Can you work these out from the model? Positions are in its coordinate system, mm. Face numbers are marked on the shaded views. Round coordinates to 2 decimals unless told otherwise and drop trailing zeros. Write each loop counter-clockwise with the first axis right and the second up, starting at its lowest first coordinate (ties: lowest second). Pieces come first, ordered by that corner, then holes. Notation, with made-up numbers: M 79.5,33.25 L 87.5,33.25 A28 cw 87.5,54.25 Z; hole C -33.5,32.5 d6. An arc over 180 degrees is marked long. Answer as a JSON object with one key per item and string values. Group by question number.
1) Please list where these lines run through material, in increasing order: L1, parallel to Z at x = 100, y = 126; L2, parallel to Y at x = 31, z = 7; L3, parallel to X at y = -38, z = 1. Write a range as [from, to].
2) Suppose I cut it at A-A, the plane z = 0. Write out the boundary of the cut face in (x, y).
3) Suppose I cut it at B-B, the plane x = 100. Write out the boundary of the cut face in (y, z).
4) If we mould it in two halves opening along Y, with no side actions, what happens to the marked faces 1, 2 and 3? For each: +Y half, -Y half, draft (parallel to the pull), parting line (faces both ways), or undercut.
5) Suppose I cut it at D-D, the plane y = 77. Write out the boundary of the cut face in (x, z).
6) I'm going to push flat-ended pins straight in: pin 1 Ø8 at (y, z) = (-5.5, -11.5) entering from -X; pin 2 Ø8 at (y, z) = (-60.5, -9.5) entering from +X (3 decimals); pin 3 Ø3 at (y, z) = (13.5, -5) entering from -X; pin 4 Ø11 at (x, z) = (100, 0) entering from +Y. Where does each tip first touch, or does it pass through?
7) Suppose I cut it at C-C, the plane x = 16. Write out the boundary of the cut face in (y, z), and give its area (3 significant figures).
from build123d import *

# Parameters (mm, degrees)
F1_R     = 6
F1_R_2   = 12.5
F2_DEPTH = 6
F3_DEPTH = 125


with BuildPart() as f2:
    # F1 (on offset) → F2 (new body)
    with BuildSketch(Plane.XZ.offset(125)):
        with BuildLine():
            Line((250, 15), (0, 15))
            ThreePointArc((0, 15), (-15, 0), (0, -15))
            Line((0, -15), (250, -15))
            ThreePointArc((250, -15), (265, 0), (250, 15))
        make_face()
        Circle(F1_R, mode=Mode.SUBTRACT)
        with Locations((100, 0)):
            Circle(F1_R, mode=Mode.SUBTRACT)
        with Locations((250, 0)):
            Circle(F1_R_2, mode=Mode.SUBTRACT)
        with Locations((250, 0)):
            Circle(F1_R_2)
    extrude(amount=F2_DEPTH)

    # F1 (on offset) → F3 (join, through all)
    with BuildSketch(Plane.XZ.offset(125)):
        with Locations((250, 0)):
            Circle(F1_R_2)
    extrude(amount=-F3_DEPTH)

    # F4: F2 across plane


with BuildPart() as f2_1:
    add(f2.part)
    add(f2.part.mirror(Plane.XZ))


solid = f2_1.part
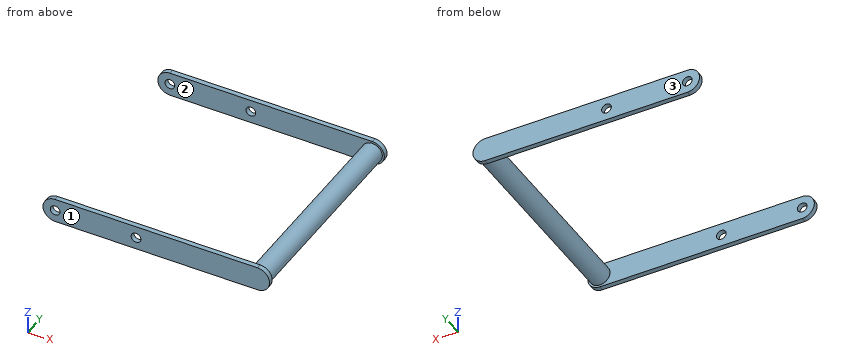
Results:
{
 "1": {"L1": "[-15, -6], [6, 15]", "L2": "[-131, -125], [125, 131]", "L3": "[237.54, 262.46]"},
 "2": {"outline": "M -15,-131 L -6,-131 L -6,-125 L -15,-125 Z; M -15,125 L -6,125 L -6,131 L -15,131 Z; M 6,-131 L 94,-131 L 94,-125 L 6,-125 Z; M 6,125 L 94,125 L 94,131 L 6,131 Z; M 106,-131 L 265,-131 L 265,-125 L 262.5,-125 L 262.5,125 L 265,125 L 265,131 L 106,131 L 106,125 L 237.5,125 L 237.5,-125 L 106,-125 Z"},
 "3": {"outline": "M -131,-15 L -125,-15 L -125,-6 L -131,-6 Z; M -131,6 L -125,6 L -125,15 L -131,15 Z; M 125,-15 L 131,-15 L 131,-6 L 125,-6 Z; M 125,6 L 131,6 L 131,15 L 125,15 Z"},
 "4": {"face 1": "-Y half", "face 2": "undercut", "face 3": "+Y half"},
 "5": {"outline": "C 250,0 d25"},
 "6": {"pin 1": "x = 240", "pin 2": "x = 261.225", "pin 3": "x = 238", "pin 4": "through"},
 "7": {"outline": "M -131,-15 L -125,-15 L -125,15 L -131,15 Z; M 125,-15 L 131,-15 L 131,15 L 125,15 Z", "area": "360 mm^2"}
}
